```python
from build123d import *

# Parameters (mm, degrees)
ESQUISSE5_R                       = 150
ESQUISSE5_R_2                     = 1.6
BASE_DEPTH                        = 5
ESQUISSE8_R                       = 1.5
FIXATION_CRAN_DEPTH               = 6
ESQUISSE9_R                       = 1.5
FIXATION_LIDAR_DEPTH              = 6
ESQUISSE7_W                       = 70
ESQUISSE7_H                       = 40
EXTRUSION_PASSAGE_DE_CABLES_DEPTH = 5
CONG_1_R                          = 6
ESQUISSE10_R                      = 1.5
EXTRUSION_FIXATION_PAROI_DEPTH    = 6
ENL_V_MAT_EXTRU_1_REACH           = 7
ESQUISSE11_R                      = 1.5


with BuildPart() as part:
    # Esquisse5 → base (new body)
    with BuildSketch(Plane.XY):
        Circle(ESQUISSE5_R)
        with Locations((99.73919487, -62.04957211)):
            Circle(ESQUISSE5_R_2, mode=Mode.SUBTRACT)
        with Locations((55.59658934, -53.636417112)):
            Circle(ESQUISSE5_R_2, mode=Mode.SUBTRACT)
        with Locations((33.380811026, -111.152193156)):
            Circle(ESQUISSE5_R_2, mode=Mode.SUBTRACT)
        with Locations((-50.043705329, -36.418231474)):
            Circle(ESQUISSE5_R_2, mode=Mode.SUBTRACT)
        with Locations((-83.063705329, 15.651768526)):
            Circle(ESQUISSE5_R_2, mode=Mode.SUBTRACT)
        with Locations((-50.043705329, 46.131768526)):
            Circle(ESQUISSE5_R_2, mode=Mode.SUBTRACT)
    extrude(amount=BASE_DEPTH)

    # Esquisse8 → fixation écran (cut, through all)
    with BuildSketch(Plane.XY.offset(5)):
        with Locations((-85.6, 63.115)):
            Circle(ESQUISSE8_R)
        with Locations((-20, 63.115)):
            Circle(ESQUISSE8_R)
        with Locations((-85.6, -63.115)):
            Circle(ESQUISSE8_R)
        with Locations((-20, -63.115)):
            Circle(ESQUISSE8_R)
    extrude(amount=-FIXATION_CRAN_DEPTH, mode=Mode.SUBTRACT)

    # Esquisse9 → fixation lidar (cut, through all)
    with BuildSketch(Plane.XY.offset(5)):
        with Locations((45, -28.5)):
            Circle(ESQUISSE9_R)
        with Locations((107, -28.5)):
            Circle(ESQUISSE9_R)
        with Locations((101, 28.5)):
            Circle(ESQUISSE9_R)
        with Locations((51, 28.5)):
            Circle(ESQUISSE9_R)
    extrude(amount=-FIXATION_LIDAR_DEPTH, mode=Mode.SUBTRACT)

    # Esquisse7 → extrusion passage de cables (cut)
    with BuildSketch(Plane.XY.offset(5)):
        with Locations((0, 90)):
            Rectangle(ESQUISSE7_W, ESQUISSE7_H)
    extrude(amount=-EXTRUSION_PASSAGE_DE_CABLES_DEPTH, mode=Mode.SUBTRACT)

    # Congé1
    cong_1_edges = [part.edges().sort_by_distance(p)[0] for p in [
        (-35, 70, 2.5),
        (-35, 110, 2.5),
        (35, 110, 2.5),
        (35, 70, 2.5),
    ]]
    fillet(cong_1_edges, radius=CONG_1_R)

    # Esquisse10 → extrusion fixation paroi (cut, through all)
    with BuildSketch(Plane.XY.offset(5)):
        with Locations((-102.530483272, 95.45941546)):
            Circle(ESQUISSE10_R)
        with Locations((-95.45941546, 102.530483272)):
            Circle(ESQUISSE10_R)
        with Locations((95.45941546, 102.530483272)):
            Circle(ESQUISSE10_R)
        with Locations((102.530483272, 95.45941546)):
            Circle(ESQUISSE10_R)
        with Locations((102.530483272, -95.45941546)):
            Circle(ESQUISSE10_R)
        with Locations((95.45941546, -102.530483272)):
            Circle(ESQUISSE10_R)
        with Locations((-95.45941546, -102.530483272)):
            Circle(ESQUISSE10_R)
        with Locations((-102.530483272, -95.45941546)):
            Circle(ESQUISSE10_R)
    extrude(amount=-EXTRUSION_FIXATION_PAROI_DEPTH, mode=Mode.SUBTRACT)

    # Esquisse11 → Enlèv. mat.-Extru.1 (cut, up to next)
    with BuildSketch(Plane.XY.offset(5), mode=Mode.PRIVATE) as enl_v_mat_extru_1_sk1:
        with Locations((-88.388347648, 109.601551084)):
            Circle(ESQUISSE11_R)
    enl_v_mat_extru_1_tool1 = extrude(enl_v_mat_extru_1_sk1.sketch, amount=-ENL_V_MAT_EXTRU_1_REACH, mode=Mode.PRIVATE) & part.part
    add(enl_v_mat_extru_1_tool1.solids().sort_by_distance((-88.388348, 109.601551, 5))[0], mode=Mode.SUBTRACT)
    # Esquisse11 → Enlèv. mat.-Extru.1 (cut, up to next)
    with BuildSketch(Plane.XY.offset(5), mode=Mode.PRIVATE) as enl_v_mat_extru_1_sk2:
        with Locations((-109.601551084, 88.388347648)):
            Circle(ESQUISSE11_R)
    enl_v_mat_extru_1_tool2 = extrude(enl_v_mat_extru_1_sk2.sketch, amount=-ENL_V_MAT_EXTRU_1_REACH, mode=Mode.PRIVATE) & part.part
    add(enl_v_mat_extru_1_tool2.solids().sort_by_distance((-109.601551, 88.388348, 5))[0], mode=Mode.SUBTRACT)
    # Esquisse11 → Enlèv. mat.-Extru.1 (cut, up to next)
    with BuildSketch(Plane.XY.offset(5), mode=Mode.PRIVATE) as enl_v_mat_extru_1_sk3:
        with Locations((-109.601551084, -88.388347648)):
            Circle(ESQUISSE11_R)
    enl_v_mat_extru_1_tool3 = extrude(enl_v_mat_extru_1_sk3.sketch, amount=-ENL_V_MAT_EXTRU_1_REACH, mode=Mode.PRIVATE) & part.part
    add(enl_v_mat_extru_1_tool3.solids().sort_by_distance((-109.601551, -88.388348, 5))[0], mode=Mode.SUBTRACT)
    # Esquisse11 → Enlèv. mat.-Extru.1 (cut, up to next)
    with BuildSketch(Plane.XY.offset(5), mode=Mode.PRIVATE) as enl_v_mat_extru_1_sk4:
        with Locations((-88.388347648, -109.601551084)):
            Circle(ESQUISSE11_R)
    enl_v_mat_extru_1_tool4 = extrude(enl_v_mat_extru_1_sk4.sketch, amount=-ENL_V_MAT_EXTRU_1_REACH, mode=Mode.PRIVATE) & part.part
    add(enl_v_mat_extru_1_tool4.solids().sort_by_distance((-88.388348, -109.601551, 5))[0], mode=Mode.SUBTRACT)
    # Esquisse11 → Enlèv. mat.-Extru.1 (cut, up to next)
    with BuildSketch(Plane.XY.offset(5), mode=Mode.PRIVATE) as enl_v_mat_extru_1_sk5:
        with Locations((88.388347648, -109.601551084)):
            Circle(ESQUISSE11_R)
    enl_v_mat_extru_1_tool5 = extrude(enl_v_mat_extru_1_sk5.sketch, amount=-ENL_V_MAT_EXTRU_1_REACH, mode=Mode.PRIVATE) & part.part
    add(enl_v_mat_extru_1_tool5.solids().sort_by_distance((88.388348, -109.601551, 5))[0], mode=Mode.SUBTRACT)
    # Esquisse11 → Enlèv. mat.-Extru.1 (cut, up to next)
    with BuildSketch(Plane.XY.offset(5), mode=Mode.PRIVATE) as enl_v_mat_extru_1_sk6:
        with Locations((109.601551084, -88.388347648)):
            Circle(ESQUISSE11_R)
    enl_v_mat_extru_1_tool6 = extrude(enl_v_mat_extru_1_sk6.sketch, amount=-ENL_V_MAT_EXTRU_1_REACH, mode=Mode.PRIVATE) & part.part
    add(enl_v_mat_extru_1_tool6.solids().sort_by_distance((109.601551, -88.388348, 5))[0], mode=Mode.SUBTRACT)
    # Esquisse11 → Enlèv. mat.-Extru.1 (cut, up to next)
    with BuildSketch(Plane.XY.offset(5), mode=Mode.PRIVATE) as enl_v_mat_extru_1_sk7:
        with Locations((109.601551084, 88.388347648)):
            Circle(ESQUISSE11_R)
    enl_v_mat_extru_1_tool7 = extrude(enl_v_mat_extru_1_sk7.sketch, amount=-ENL_V_MAT_EXTRU_1_REACH, mode=Mode.PRIVATE) & part.part
    add(enl_v_mat_extru_1_tool7.solids().sort_by_distance((109.601551, 88.388348, 5))[0], mode=Mode.SUBTRACT)
    # Esquisse11 → Enlèv. mat.-Extru.1 (cut, up to next)
    with BuildSketch(Plane.XY.offset(5), mode=Mode.PRIVATE) as enl_v_mat_extru_1_sk8:
        with Locations((88.388347648, 109.601551084)):
            Circle(ESQUISSE11_R)
    enl_v_mat_extru_1_tool8 = extrude(enl_v_mat_extru_1_sk8.sketch, amount=-ENL_V_MAT_EXTRU_1_REACH, mode=Mode.PRIVATE) & part.part
    add(enl_v_mat_extru_1_tool8.solids().sort_by_distance((88.388348, 109.601551, 5))[0], mode=Mode.SUBTRACT)


solid = part.part
```
Input: part model. Units: mm. Frame: model coordinates. Give positions to 0.01 mm unless a question says otherwise; leave off trailing zeros. Order: outer loops, then holes, each group sorted by start corner. A loop starts at its lowest first (then second) coordinate and runs counter-clockwise, first axis right, second up. Notation, with made-up numbers: (17.5, 61.25) - (65.5, 61.25) arc R5 cw to (65.5, 65.25) - close; hole circle Ø3 at (87, 72.5). An arc over 180 degrees is marked (long way). Put each result on its own line as item: value.
Item 1: Section query B-B, the plane z = 1.7. Count the separate pieces of the cut face and the enclosed holes in it, then the cut area to 3 significant figures.
Found:
separate pieces: 1
enclosed holes: 31
area: 67,700 mm^2
Item 2: Contact query for flat-ended pins moving along their axis: pin 1 (3 mm diameter, centred on x = 57.5, z = 2.5, fed in from -Y); pin 2 (2.5 mm diameter, centred on x = 107, y = -28.5, fed in from -Z). Output: stop coordinate, or through.
Found:
pin 1: stops at y = -139.15
pin 2: passes through
Item 3: Ray query, L1, parallel to Y at x = -20, z = 3.4 (3 decimals); L2, parallel to Y at x = -109, z = 4.1; L3, parallel to X at y = 80, z = 2.3. Return the intervals inside material, ascending. Write a range as from..to.
Found:
L1: y = -148.661..-64.615, -61.615..61.615, 64.615..70, 110..148.661
L2: y = -103.05..-89.76, -87.01..87.01, 89.76..103.05
L3: x = -126.89..-35, 35..126.89
Item 4: Section query C-C, the plane y = -116.5. Return loops of the section in (x, z), then the cut area to 3 significant figures.
Found:
outline: (-94.49, 0) - (94.49, 0) - (94.49, 5) - (-94.49, 5) - close
area: 945 mm^2
Item 5: Draft query along X for faces 1 (the flat face through (-2, 2, 5)), 2 (the cylindrical face through (-19.527, 148.724, 2.465)). Return one class per face: +X half, -X half, draft (parallel to the pull), parting line (faces both ways), or undercut.
Found:
face 1: draft
face 2: parting line
Item 6: Section query A-A, the plane y = -46.5. Return loops of the section in (x, z), then the cut area to 3 significant figures.
Found:
outline: (-142.61, 0) - (142.61, 0) - (142.61, 5) - (-142.61, 5) - close
area: 1,430 mm^2
